from build123d import *

# Parameters (mm, degrees)
SKETCH1_R           = 2.5527
BOSS_EXTRUDE1_DEPTH = 3.175


with BuildPart() as part:
    # Sketch1 → Boss-Extrude1 (new body)
    with BuildSketch(Plane(origin=(0, 0, 0), x_dir=(-1, 0, 0), z_dir=(0, 0, -1))):
        with BuildLine():
            Line((-2.414213562, 0.585786438), (-0.585786438, 2.414213562))
            ThreePointArc((-0.585786438, 2.414213562), (-0.152240935, 3.06306026), (0, 3.828427125))
            Line((0, 3.828427125), (0, 72.371572875))
            ThreePointArc((0, 72.371572875), (-0.152240935, 73.13693974), (-0.585786438, 73.785786438))
            Line((-0.585786438, 73.785786438), (-2.414213562, 75.614213562))
            ThreePointArc((-2.414213562, 75.614213562), (-3.06306026, 76.047759065), (-3.828427125, 76.2))
            Line((-3.828427125, 76.2), (-21.571572875, 76.2))
            ThreePointArc((-21.571572875, 76.2), (-22.33693974, 76.047759065), (-22.985786438, 75.614213562))
            Line((-22.985786438, 75.614213562), (-24.814213562, 73.785786438))
            ThreePointArc((-24.814213562, 73.785786438), (-25.247759065, 73.13693974), (-25.4, 72.371572875))
            Line((-25.4, 72.371572875), (-25.4, 62.502257193))
            ThreePointArc((-25.4, 62.502257193), (-25.615298321, 61.050833807), (-26.242651938, 59.724406028))
            Line((-26.242651938, 59.724406028), (-30.100625257, 53.950540928))
            ThreePointArc((-30.100625257, 53.950540928), (-31.086006897, 52.863339826), (-32.344556156, 52.10899443))
            Line((-32.344556156, 52.10899443), (-75.296592814, 34.317678315))
            ThreePointArc((-75.296592814, 34.317678315), (-76.719924274, 33.961152344), (-78.185461586, 34.033149576))
            Line((-78.185461586, 34.033149576), (-84.996199847, 35.387889647))
            ThreePointArc((-84.996199847, 35.387889647), (-86.377731921, 35.882209727), (-87.556282143, 36.756282143))
            Line((-87.556282143, 36.756282143), (-94.534942187, 43.734942187))
            ThreePointArc((-94.534942187, 43.734942187), (-95.183788885, 44.16848769), (-95.94915575, 44.320728625))
            Line((-95.94915575, 44.320728625), (-98.534942187, 44.320728625))
            ThreePointArc((-98.534942187, 44.320728625), (-99.300309052, 44.16848769), (-99.94915575, 43.734942187))
            Line((-99.94915575, 43.734942187), (-112.49545443, 31.188643508))
            ThreePointArc((-112.49545443, 31.188643508), (-112.928999932, 30.53979681), (-113.081240867, 29.774429945))
            Line((-113.081240867, 29.774429945), (-113.081240867, 27.188643508))
            ThreePointArc((-113.081240867, 27.188643508), (-112.928999932, 26.423276643), (-112.49545443, 25.774429945))
            Line((-112.49545443, 25.774429945), (-64.028131265, -22.692893219))
            ThreePointArc((-64.028131265, -22.692893219), (-63.379284568, -23.126438721), (-62.613917703, -23.278679656))
            Line((-62.613917703, -23.278679656), (-60.028131265, -23.278679656))
            ThreePointArc((-60.028131265, -23.278679656), (-59.262764401, -23.126438721), (-58.613917703, -22.692893219))
            Line((-58.613917703, -22.692893219), (-44.063773661, -8.142749177))
            ThreePointArc((-44.063773661, -8.142749177), (-43.30609092, -7.520935021), (-42.441656917, -7.05888542))
            Line((-42.441656917, -7.05888542), (-26.318855325, -0.380602337))
            ThreePointArc((-26.318855325, -0.380602337), (-25.380889773, -0.096073598), (-24.405438163, 0))
            Line((-24.405438163, 0), (-3.828427125, 0))
            ThreePointArc((-3.828427125, 0), (-3.06306026, 0.152240935), (-2.414213562, 0.585786438))
        make_face()
        with Locations((-29.720392856, 9.920375508)):
            Circle(SKETCH1_R, mode=Mode.SUBTRACT)
        with Locations((-47.32029795, 2.630256121)):
            Circle(SKETCH1_R, mode=Mode.SUBTRACT)
        with Locations((-12.7, 12.7)):
            Circle(SKETCH1_R, mode=Mode.SUBTRACT)
        with Locations((-12.7, 38.1)):
            Circle(SKETCH1_R, mode=Mode.SUBTRACT)
        with Locations((-12.7, 63.5)):
            Circle(SKETCH1_R, mode=Mode.SUBTRACT)
        with Locations((-12.7, 25.4)):
            Circle(SKETCH1_R, mode=Mode.SUBTRACT)
        with Locations((-12.7, 50.8)):
            Circle(SKETCH1_R, mode=Mode.SUBTRACT)
        with Locations((-70.301280605, 1.540768363)):
            Circle(SKETCH1_R, mode=Mode.SUBTRACT)
        with Locations((-88.261792847, 19.501280605)):
            Circle(SKETCH1_R, mode=Mode.SUBTRACT)
        with Locations((-97.242048969, 28.481536726)):
            Circle(SKETCH1_R, mode=Mode.SUBTRACT)
        with Locations((-79.281536726, 10.521024484)):
            Circle(SKETCH1_R, mode=Mode.SUBTRACT)
        with Locations((-61.321024484, -7.439487758)):
            Circle(SKETCH1_R, mode=Mode.SUBTRACT)
        with Locations((-37.010512242, 27.520280602)):
            Circle(SKETCH1_R, mode=Mode.SUBTRACT)
        with Locations((-54.610417336, 20.230161215)):
            Circle(SKETCH1_R, mode=Mode.SUBTRACT)
        with Locations((-42.165405096, 15.075268362)):
            Circle(SKETCH1_R, mode=Mode.SUBTRACT)
        with Locations((-37.010512242, 2.630256121)):
            Circle(SKETCH1_R, mode=Mode.SUBTRACT)
        with BuildLine():
            Line((-49.678685233, 26.543404604), (-51.813911765, 31.698297458))
            ThreePointArc((-51.813911765, 31.698297458), (-50.43240048, 35.033560738), (-47.0971372, 33.652049454))
            Line((-47.0971372, 33.652049454), (-44.961910667, 28.4971566))
            ThreePointArc((-44.961910667, 28.4971566), (-46.343421952, 25.161893319), (-49.678685233, 26.543404604))
        make_face(mode=Mode.SUBTRACT)
    extrude(amount=-BOSS_EXTRUDE1_DEPTH)


solid = part.part
Source: CAD feature listing. Evaluate the final solid. Frame: model axes, mm. A direction names the side the tool comes from. Round coordinates to 2 decimals unless told otherwise and drop trailing zeros. Loops run counter-clockwise (first coordinate to the right, second up) from the corner with the lowest first, then second, coordinate; pieces in that order, holes last. Notation, with made-up numbers: (75, 68) - (125, 68) arc R17 cw to (125, 81) - close; hole circle Ø8 at (-34.5, 59.5). An arc over 180 degrees is marked (long way). Write item = value, one per line. Start each with the question number.
Item 1: Reachability of faces 1 (the face through (25.4, 68, 2)), 2 (the face through (50.73, 29.08, 1.57)), 3 (the face through (81.54, 34.7, 1.57)), 4 (the face through (0, 38, 2)) from +Z, -Z, +X, -X, +Y, -Y: full face, straight path, thin tool, end or side. Return the list, or none.
Item 2: Material intervals for line 1 (Y direction, x = 12.7, z = 1.85); line 2 (X direction, y = 27, z = 0.9); line 3 (X direction, y = 15, z = 1.65), sorted ascending.
Item 3: Section query B-B on y = 50.8. Output: boundary loops of the cut face in (x, z) (3 decimals), plus the area to 3 significant figures.
Item 4: Mould query, pull axis Y, two halves, no side actions, for faces 5 (the face through (61, -23.279, 2)), 6 (the face through (45, 16, 0)), 7 (the face through (46, 31, 2)). Classes: released by +Y, released by -Y, zero draft, split by the parting line, or undercut.
Item 5: Section query D-D on y = -14. Output: boundary loops of the cut face in (x, z) (3 decimals).
Item 6: Section query A-A on x = 69. Output: boundary loops of the cut face in (y, z) (3 decimals), plus the area to 3 significant figures.
Item 7: First-contact query: pin 1 Ø1 at (y, z) = (21, 0.5) entering from +X; pin 2 Ø1.3 at (x, z) = (97.5, 2) entering from +Y; pin 3 Ø1.5 at (x, z) = (70.5, 2.5) entering from -Y. Flat tips, straight axial feed; report the tip coordinate or a pass-through.
Item 8: Section query C-C on z = 0.85. Count the separate pieces of the cut face and the enclosed holes in it, plus the area to 3 significant figures.
Results list:
q1.face_1 = +Z, -Z, +X, +Y
q1.face_2 = +Z, -Z
q1.face_3 = +Z, -Z, +Y
q1.face_4 = +Z, -Z, -X, +Y, -Y
q2.line_1 = 0 to 10.15, 15.25 to 22.85, 27.95 to 35.55, 40.65 to 48.25, 53.35 to 60.95, 66.05 to 76.2
q2.line_2 = 0 to 10.71, 14.69 to 34.51, 39.51 to 44.82, 49.87 to 95.16, 99.32 to 113.07
q2.line_3 = 0 to 11.59, 13.81 to 39.61, 44.72 to 101.72
q3.outline = (0, 0) - (10.147, 0) - (10.147, 3.175) - (0, 3.175) - close; (15.253, 0) - (35.505, 0) - (35.505, 3.175) - (15.253, 3.175) - close
q3.area = 96.5 mm²
q4.face_5 = released by -Y
q4.face_6 = zero draft
q4.face_7 = undercut
q5.outline = (49.921, 0) - (72.721, 0) - (72.721, 3.175) - (49.921, 3.175) - close
q6.outline = (-17.721, 0) - (-0.655, 0) - (-0.655, 3.175) - (-17.721, 3.175) - close; (3.737, 0) - (36.926, 0) - (36.926, 3.175) - (3.737, 3.175) - close
q6.area = 160 mm²
q7.pin_1 = 108.22
q7.pin_2 = 44.32
q7.pin_3 = -16.97
q8.separate_pieces = 1
q8.enclosed_holes = 17
q8.area = 5,560 mm²
